from build123d import *

# Parameters (mm, degrees)
F1_DEPTH        = 12.7
F5_DEPTH        = 20.32
F4_W            = 63.5
F4_H            = 38.1
F9_D            = 12.7
F11_D           = 4.826
F11_CBORE_D     = 9.4742
F11_CBORE_DEPTH = 3.3782
F12_R           = 2.54


with BuildPart() as f1:
    # F0 (on Front) → F1 (new body)
    with BuildSketch(Plane.XZ):
        with BuildLine():
            ThreePointArc((0, 19.05), (5.5796158184, 5.5796158184), (19.05, 0))
            Line((19.05, 0), (82.55, 0))
            ThreePointArc((82.55, 0), (96.0203841816, 5.5796158184), (101.6, 19.05))
            ThreePointArc((101.6, 19.05), (96.0203841816, 32.5203841816), (82.55, 38.1))
            Line((82.55, 38.1), (19.05, 38.1))
            ThreePointArc((19.05, 38.1), (5.5796158184, 32.5203841816), (0, 19.05))
        make_face()
    extrude(amount=F1_DEPTH)


with BuildPart() as f5:
    # F3 (on offset) → F5 (new body)
    with BuildSketch(Plane.XZ.offset(93.98)):
        with BuildLine():
            ThreePointArc((22.86, 19.05), (26.5797438789, 10.0697438789), (35.56, 6.35))
            Line((35.56, 6.35), (66.04, 6.35))
            ThreePointArc((66.04, 6.35), (75.0202561211, 10.0697438789), (78.74, 19.05))
            ThreePointArc((78.74, 19.05), (75.0202561211, 28.0302561211), (66.04, 31.75))
            Line((66.04, 31.75), (35.56, 31.75))
            ThreePointArc((35.56, 31.75), (26.5797438789, 28.0302561211), (22.86, 19.05))
        make_face()
    extrude(amount=F5_DEPTH)


with BuildPart() as f6:
    # F4 (on face) → F6 section 0
    with BuildSketch(Plane.XZ.offset(12.7)):
        with Locations((50.8, 19.05)):
            Rectangle(F4_W, F4_H)
    # F5_face (on face) → F6 section 1
    with BuildSketch(Plane(origin=(50.8, -93.98, 19.05), x_dir=(1, 0, 0), z_dir=(0, 1, 0))):
        with BuildLine():
            ThreePointArc((-15.24, 12.7), (-27.94, 0), (-15.24, -12.7))
            Line((-15.24, -12.7), (15.24, -12.7))
            ThreePointArc((15.24, -12.7), (27.94, 0), (15.24, 12.7))
            Line((15.24, 12.7), (-15.24, 12.7))
        make_face()
    loft()


with BuildPart() as f1_1:
    add(f1.part)

    # F7: union F5, F6
    add(f5.part)
    add(f6.part)

    # F9 (through all)
    with Locations(Plane.XY.offset(31.75)):
        with Locations((50.8, -104.14)):
            Hole(F9_D / 2)

    # F11 (through all)
    with Locations(Plane.XZ.offset(12.7)):
        with Locations((9.525, 19.05), (92.075, 19.05)):
            CounterBoreHole(F11_D / 2, F11_CBORE_D / 2, F11_CBORE_DEPTH)

    # F12
    f12_edges = [f1_1.edges().sort_by_distance(p)[0] for p in [
        (50.8, -114.3, 31.75),
    ]]
    fillet(f12_edges, radius=F12_R)


solid = f1_1.part
Check sheet for the modelled part. Datum: model origin and axes. Units: mm. A direction names the side the tool comes from. Coordinates: 2 decimals unless noted, no trailing zeros. Write each loop counter-clockwise with the first axis right and the second up, starting at its lowest first coordinate (ties: lowest second). Pieces come first, ordered by that corner, then holes.
Item 1: Depth check by flat-ended pin: pin 1 Ø9.5 at (x, z) = (9.5, 19) entering from -Y; pin 2 Ø9 at (x, y) = (52.5, -103) entering from -Z; pin 3 Ø4 at (x, y) = (25, -77.5) entering from -Z. Enter the tip coordinate at first touch or a pass-through.
Numbers:
pin 1: stops at y = -12.7
pin 2: stops at z = 6.35
pin 3: stops at z = 7.82
Item 2: Cross-section at A-A on y = -104.14. Record the boundary of the cut face in (x, z), then the cut area to 3 significant figures.
Numbers:
outline: (35.56, 6.35) - (44.45, 6.35) - (44.45, 31.75) - (35.56, 31.75) arc R12.7 ccw to start; (57.15, 6.35) - (66.04, 6.35) arc R12.7 ccw to (66.04, 31.75) - (57.15, 31.75) - close
area: 958 mm2
Item 3: Mould release check, pull along Z, two halves, no side actions. Record for faces 1 (the face through (11.44, -4.6, 17.58)), 2 (the face through (50, 0, 19)), 3 (the face through (51, -97, 6.35)): released by +Z, released by -Z, zero draft, split by the parting line, or undercut.
Numbers:
face 1: undercut
face 2: zero draft
face 3: released by -Z
Item 4: Scan lines: probe 1 along Y at (x, z) = (11, 13); probe 2 along Y at (x, z) = (50.8, 24.75); probe 3 along Y at (x, z) = (94.5, 16.5). Record each from-to range of solid material in increasing order.
Numbers:
probe 1: y = -12.7 to 0
probe 2: y = -114.3 to -110.49, -97.79 to 0
probe 3: y = -9.32 to 0
Item 5: Access from +Z, -Z, +X, -X, +Y, -Y to the whole of each face (thin tool, end or side, straight path). Record for faces 4 (the face through (7, -9.322, 20)), 5 (the face through (12, -12.7, 24)), 6 (the face through (90, -12.7, 24)).
Numbers:
face 4: -Y
face 5: +Z, -Z, -X, -Y
face 6: +Z, -Z, +X, -Y
